Design review of the part built by this model. Coordinates are the model's own, in mm. A direction names the side the tool comes from. Give positions to 0.01 mm unless a question says otherwise; leave off trailing zeros. Loops run counter-clockwise (first coordinate to the right, second up) from the corner with the lowest first, then second, coordinate; pieces in that order, holes last. Notation, with made-up numbers: (38.5, 87.25) -> (97.5, 87.25) arc R16 cw to (97.5, 101.25) -> close; hole circle Ø1 at (54, 2.5). An arc over 180 degrees is marked (long way). Answer as CSV lines item,"result".
from build123d import *

# Parameters (mm, degrees)
BOSS_EXTRUDE1_DEPTH = 1.75
FILLET1_R           = 1
FILLET2_R           = 1.5
FILLET3_R           = 2
FILLET4_R           = 2.5
FILLET5_R           = 3
FILLET6_R           = 4
FILLET7_R           = 16.3
CUT_EXTRUDE1_REACH  = 152.576
SKETCH4_R           = 17.447294951


with BuildPart() as part:
    # Sketch1 → Boss-Extrude1 (new body)
    with BuildSketch(Plane.XZ.offset(122.00000003)):
        Polygon((0, -17.251221002), (25.25, -8.499999866), (25.25, 9.000000134), (0, 17.122631398), (-25.25, 9.000000134), (-25.25, -8.499999866), align=None)
    extrude(amount=-BOSS_EXTRUDE1_DEPTH)

    # Sketch2 → Revolve1 (revolve)
    with BuildSketch(Plane(origin=(0, 0, 0), x_dir=(-1, 0, 0), z_dir=(0, 0, -1)), mode=Mode.PRIVATE) as revolve1_sk:
        Polygon((-15.000000104, -120.25000003), (0, -120.25000003), (0, 50.000000745), (-3.000000045, 50.000000745), (-4.510515864, 25.545941813), (-5.250000063, 25.308142899), (-5.250000063, 12.808142939), (-15.000000104, 8.474809587), align=None)
    revolve(revolve1_sk.sketch.rotate(Axis((0, -120.25000003, 0), (0, 1, 0)), 270), axis=Axis((0, -120.25000003, 0), (0, 1, 0)))

    # Sketch3 → Cut-Revolve1 (revolve, cut)
    with BuildSketch(Plane(origin=(0, 0, 0), x_dir=(-1, 0, 0), z_dir=(0, 0, -1)), mode=Mode.PRIVATE) as cut_revolve1_sk:
        Polygon((-14.00000011, -122.00000003), (0, -122.00000003), (0, 50.000000745), (-1.700000001, 50.000000745), (-4.165865434, 12.195663018), (-14.00000011, 7.824936496), align=None)
    revolve(cut_revolve1_sk.sketch.rotate(Axis((0, -122.00000003, 0), (0, 1, 0)), 90), axis=Axis((0, -122.00000003, 0), (0, 1, 0)), mode=Mode.SUBTRACT)

    # Fillet1
    fillet1_edges = [part.edges().sort_by_distance(p)[0] for p in [
        (0, 50.000000745, -3.000000045),
    ]]
    fillet(fillet1_edges, radius=FILLET1_R)

    # Fillet2
    fillet2_edges = [part.edges().sort_by_distance(p)[0] for p in [
        (0, 7.824936496, 14.00000011),
    ]]
    fillet(fillet2_edges, radius=FILLET2_R)

    # Fillet3
    fillet3_edges = [part.edges().sort_by_distance(p)[0] for p in [
        (-25.25, -121.12500003, -8.499999866),
        (-25.25, -121.12500003, 9.000000134),
        (25.25, -121.12500003, 9.000000134),
        (25.25, -121.12500003, -8.499999866),
    ]]
    fillet(fillet3_edges, radius=FILLET3_R)

    # Fillet4
    fillet4_edges = [part.edges().sort_by_distance(p)[0] for p in [
        (0, 8.474809587, -15.000000104),
    ]]
    fillet(fillet4_edges, radius=FILLET4_R)

    # Fillet5
    fillet5_edges = [part.edges().sort_by_distance(p)[0] for p in [
        (0, 12.808142939, -5.250000063),
    ]]
    fillet(fillet5_edges, radius=FILLET5_R)

    # Fillet6
    fillet6_edges = [part.edges().sort_by_distance(p)[0] for p in [
        (0, 12.195663018, 4.165865434),
    ]]
    fillet(fillet6_edges, radius=FILLET6_R)

    # Fillet7
    fillet7_edges = [part.edges().sort_by_distance(p)[0] for p in [
        (0, -121.12500003, 17.122631398),
        (0, -121.12500003, -17.251221002),
    ]]
    fillet(fillet7_edges, radius=FILLET7_R)

    # Sketch4 → Cut-Extrude1 (cut, up to next)
    with BuildSketch(Plane(origin=(0, 25.545941813, 0), x_dir=(-1, 0, 0), z_dir=(0, -1, 0)), mode=Mode.PRIVATE) as cut_extrude1_sk1:
        Circle(SKETCH4_R)
    cut_extrude1_tool1 = extrude(cut_extrude1_sk1.sketch, amount=-CUT_EXTRUDE1_REACH, mode=Mode.PRIVATE) & part.part
    add(cut_extrude1_tool1.solids().sort_by_distance((0, 25.545942, 0))[0], mode=Mode.SUBTRACT)


solid = part.part
Q1. For faces 1 (the cylindrical face through (5.205, 19.959, -0.683)), 2 (the cylindrical face through (8.52, -58.48, 11.11)), 3 (the flat face through (-14.295, -121.137, 12.524)), list the 3-axis set-ups (+Z, -Z, +X, -X, +Y, -Y) from which the entire face can be reached by the end or side of a thin tool; tool diameter is ignored.
Filled sheet:
face 1,"+Y"
face 2,"-Y"
face 3,"+Z, -X, +Y, -Y"
Q2. We need section B-B, the plane x = -21. State the section outline as (y, z) points, and give its area (3 significant figures).
Filled sheet:
outline,"(-122, -9.97) -> (-120.25, -9.97) -> (-120.25, 10.37) -> (-122, 10.37) -> close"
area,"35.6 mm^2"
Q3. Clearance check with flat-ended pins moving along their axes: pin 1 Ø3 at (x, y) = (-12.5, -56) entering from -Z; pin 2 Ø4 at (x, z) = (-13.5, -11) entering from +Y; pin 3 Ø1 at (x, z) = (-12.5, -2) entering from -Y. State where each tip first meets the part, or that it passes through.
Filled sheet:
pin 1,"stops at z = -10.2"
pin 2,"stops at y = -120.25"
pin 3,"stops at y = 8.2"
Q4. The part is to be moulded in two halves that separate along X. For faces 4 (the conical face through (3.244, 20.001, -1.687)), 5 (the flat face through (14.56, -121.14, 12.44)), 6 (the cylindrical face through (-9, -58, -12)), say which applies: pulls with the +X half, pulls with the -X half, needs draft (parallel to the pull), parting line crosses it, or undercut.
Filled sheet:
face 4,"undercut"
face 5,"pulls with the +X half"
face 6,"parting line crosses it"
Q5. To check wall thickness, follow probe 1 along X at (y, z) = (-73, 0); probe 2 along Y at (x, z) = (17.5, -6.5); probe 3 along Z at (x, y) = (3, -44). State the ranges of each line that lie inside material, in increasing order. Write a range as from..to.
Filled sheet:
probe 1,"x = -15..-14, 14..15"
probe 2,"y = -122..-120.25"
probe 3,"z = -14.7..-13.67, 13.67..14.7"
Q6. We need section A-A, the plane y = -107. State the section outline as (x, z) points, and give its area (3 significant figures).
Filled sheet:
outline,"circle Ø30 at (0, 0); hole circle Ø28 at (0, 0)"
area,"91.1 mm^2"
